CAD build for the part. Positions are in the model's coordinates, mm. A direction names the side the tool comes from. Give positions to 0.01 mm unless a question says otherwise; leave off trailing zeros. Order: outer loops, then holes, each group sorted by start corner. A loop starts at its lowest first (then second) coordinate and runs counter-clockwise, first axis right, second up. Notation, with made-up numbers: M -18.75,42.5 L 22.25,42.5 A9 cw 22.25,51.5 Z; hole C 78,59.25 d2. An arc over 180 degrees is marked long. Put each result on its own line as item: value. Start each with the question number.
1) Cut at A-A (z = -17). Write the cut outline in (x, y), and give its area (3 significant figures).
2) Cut at C-C (y = 4). Give the number of separate pieces and of enclosed holes in the cut face, and give its area (3 significant figures).
3) Cut at B-B (x = 14). Write the cut outline in (y, z), and give its area (3 significant figures).
4) Tool access for faces 1 (the face through (-6.8, 4.7, 12.9)), 2 (the face through (-12.9, 4.7, 6.8)), 3 (the face through (-15.5, 4.8, 12)), 4 (the face through (9.3, 4.8, -13.9)), 5 (the face through (12.6, 4.7, -6.8)): list every direction of +Z, -Z, +X, -X, +Y, -Y with a clear straight run to the whole face (end or side of a thin tool).
5) Pin check, flat tips, straight feed: pin 1 (1.5 mm diameter, centred on x = 15, z = 14.5, fed in from +Y); pin 2 (1 mm diameter, centred on y = 5, z = -11.5, fed in from -X); pin 3 (2.5 mm diameter, centred on y = 5.5, z = 19, fed in from -X). Stop position of each tip, or through.
6) Two-plate mould, pull along Z, no slides. Class faces 6 (the face through (-14, 3.5, 14)), 7 (the face through (18.7, 4.8, 14.1)), 8 (the face through (13.9, 4.8, -18.7)): released by +Z, released by -Z, zero draft, split by the parting line, or undercut.
7) Drill centre lines: line 1 (X direction, y = 4, z = -15); line 2 (Z direction, x = -12, y = 4.5); line 3 (Z direction, x = -10.5, y = 4.75). Where is each one in solid material? Low to high. Write a range as [from, to].
8) Cut at D-D (z = -12.5). Write the cut outline in (x, y), and give its area (3 significant figures).
```python
from build123d import *

# Parameters (mm, degrees)
SKETCH1_W               = 40
SKETCH1_H               = 40
BOSS_EXTRUDE1_DEPTH     = 6
SKETCH2_W               = 12
SKETCH2_H               = 12
CUT_EXTRUDE1_DEPTH      = 2.5
CHAMFER1_SIZE           = 2.5
SKETCH3_W               = 12
SKETCH3_H               = 12
BOSS_EXTRUDE2_DEPTH     = 2.5
CHAMFER2_SIZE           = 2.5
CIRPATTERN1_OUTLINE_W   = 7
CIRPATTERN1_OUTLINE_H   = 7
CIRPATTERN1_DEPTH       = 2.5
CIRPATTERN1_DRAFT       = 45
CIRPATTERN1_2_OUTLINE_W = 7
CIRPATTERN1_2_OUTLINE_H = 7
CIRPATTERN1_2_DEPTH     = 2.5
CIRPATTERN1_2_DRAFT     = 45
CIRPATTERN1_3_OUTLINE_W = 7
CIRPATTERN1_3_OUTLINE_H = 7
CIRPATTERN1_3_DEPTH     = 2.5
CIRPATTERN1_3_DRAFT     = 45
SKETCH4_R               = 2.5
CUT_EXTRUDE2_DEPTH      = 2.5
CIRPATTERN2_COUNT       = 4


# Read off the part's stored shape, not the designer's step: CirPattern1
# Some blends are built 0.0001 mm under size
with BuildPart() as part:
    # Sketch1 → Boss-Extrude1 (new body)
    with BuildSketch(Plane(origin=(0, 0, 0), x_dir=(1, 0, 0), z_dir=(0, 1, 0))):
        Rectangle(SKETCH1_W, SKETCH1_H)
    extrude(amount=BOSS_EXTRUDE1_DEPTH)

    # Sketch2 → Cut-Extrude1 (cut)
    with BuildSketch(Plane(origin=(0, 6, 0), x_dir=(1, 0, 0), z_dir=(0, 1, 0))):
        with Locations((14, 14)):
            Rectangle(SKETCH2_W, SKETCH2_H)
        with Locations((-14, 14)):
            Rectangle(SKETCH2_W, SKETCH2_H)
        with Locations((14, -14)):
            Rectangle(SKETCH2_W, SKETCH2_H)
        with Locations((-14, -14)):
            Rectangle(SKETCH2_W, SKETCH2_H)
    extrude(amount=-CUT_EXTRUDE1_DEPTH, mode=Mode.SUBTRACT)

    # Chamfer1
    chamfer1_edges = [part.edges().sort_by_distance(p)[0] for p in [
        (-20, 6, 0),
        (-14, 6, -8),
        (-8, 6, -14),
        (0, 6, -20),
        (8, 6, -14),
        (14, 6, -8),
        (20, 6, 0),
        (14, 6, 8),
        (8, 6, 14),
        (0, 6, 20),
        (-8, 6, 14),
        (-14, 6, 8),
    ]]
    chamfer(chamfer1_edges, length=CHAMFER1_SIZE - 0.0001)  # a hair under: the kernel refuses the full size

    # Sketch3 → Boss-Extrude2 (add)
    with BuildSketch(Plane(origin=(0, 3.5, 0), x_dir=(1, 0, 0), z_dir=(0, 1, 0))):
        with Locations((-14, -14)):
            Rectangle(SKETCH3_W, SKETCH3_H)
    extrude(amount=BOSS_EXTRUDE2_DEPTH)

    # Chamfer2
    # the kernel refuses this chamfer: 2.5 mm, written as the material it takes off along each edge
    with BuildSketch(Plane(origin=(-26.42920747, 6, 8), x_dir=(0, -0.9996219169112968, -0.027495876610586317), z_dir=(1, 0, 0)), Plane(origin=(-8, 6, 8), x_dir=(0.027495876610586317, -0.9996219169112968, 0), z_dir=(0, 0, 1))) as chamfer2_piece_1:
        Polygon((CHAMFER2_SIZE * 0.999621916911, -CHAMFER2_SIZE * 0.0274958766106), (-CHAMFER2_SIZE * 0.0274958766106, -CHAMFER2_SIZE * 0.999621916911), (0, 0), align=None)
    extrude(amount=18.42920747, mode=Mode.SUBTRACT)
    with BuildSketch(Plane(origin=(-1.57079253, 6, 20), x_dir=(0, -0.9996219169112968, 0.027495876610586317), z_dir=(-1, 0, 0))) as chamfer2_piece_2:
        Polygon((CHAMFER2_SIZE * 0.999621916911, -CHAMFER2_SIZE * 0.0274958766106), (-CHAMFER2_SIZE * 0.0274958766106, -CHAMFER2_SIZE * 0.999621916911), (0, 0), align=None)
    extrude(amount=24.85841494, mode=Mode.SUBTRACT)
    with BuildSketch(Plane(origin=(-20, 6, 26.42920747), x_dir=(0.9996219169112968, 0.027495876610586317, 0), z_dir=(0, 0, -1))) as chamfer2_piece_3:
        Polygon((CHAMFER2_SIZE * 0.999621916911, CHAMFER2_SIZE * 0.0274958766106), (-CHAMFER2_SIZE * 0.0274958766106, CHAMFER2_SIZE * 0.999621916911), (0, 0), align=None)
    extrude(amount=24.85841494, mode=Mode.SUBTRACT)


with BuildPart() as cirpattern1_tool:
    # CirPattern1 outline → CirPattern1 (with draft: the straight prism first)
    with BuildSketch(Plane(origin=(0, 6, 0), x_dir=(1, 0, 0), z_dir=(0, 1, 0))):
        with Locations((14, -14)):
            Rectangle(CIRPATTERN1_OUTLINE_W, CIRPATTERN1_OUTLINE_H)
    extrude(amount=-CIRPATTERN1_DEPTH)
    # CirPattern1: the draft: its side faces are tilted about the plane it starts from
    cirpattern1_sides = [cirpattern1_tool.faces().sort_by_distance(p)[0] for p in [
        (14, 4.75, 10.5),
        (10.5, 4.75, 14),
        (14, 4.75, 17.5),
        (17.5, 4.75, 14),
    ]]
    draft(cirpattern1_sides, Plane(origin=(0, 6, 0), x_dir=(1, 0, 0), z_dir=(0, 1, 0)), CIRPATTERN1_DRAFT)


with BuildPart() as part_1:
    add(part.part)

    # CirPattern1: add cirpattern1_tool
    add(cirpattern1_tool.part)


with BuildPart() as cirpattern1_2_tool:
    # CirPattern1 2 outline → CirPattern1 2 (with draft: the straight prism first)
    with BuildSketch(Plane(origin=(0, 6, 0), x_dir=(1, 0, 0), z_dir=(0, 1, 0))):
        with Locations((14, 14)):
            Rectangle(CIRPATTERN1_2_OUTLINE_W, CIRPATTERN1_2_OUTLINE_H)
    extrude(amount=-CIRPATTERN1_2_DEPTH)
    # CirPattern1 2: the draft: its side faces are tilted about the plane it starts from
    cirpattern1_2_sides = [cirpattern1_2_tool.faces().sort_by_distance(p)[0] for p in [
        (10.5, 4.75, -14),
        (14, 4.75, -10.5),
        (17.5, 4.75, -14),
        (14, 4.75, -17.5),
    ]]
    draft(cirpattern1_2_sides, Plane(origin=(0, 6, 0), x_dir=(1, 0, 0), z_dir=(0, 1, 0)), CIRPATTERN1_2_DRAFT)


with BuildPart() as part_2:
    add(part_1.part)

    # CirPattern1 2: add cirpattern1_2_tool
    add(cirpattern1_2_tool.part)


with BuildPart() as cirpattern1_3_tool:
    # CirPattern1 3 outline → CirPattern1 3 (with draft: the straight prism first)
    with BuildSketch(Plane(origin=(0, 6, 0), x_dir=(1, 0, 0), z_dir=(0, 1, 0))):
        with Locations((-14, 14)):
            Rectangle(CIRPATTERN1_3_OUTLINE_W, CIRPATTERN1_3_OUTLINE_H)
    extrude(amount=-CIRPATTERN1_3_DEPTH)
    # CirPattern1 3: the draft: its side faces are tilted about the plane it starts from
    cirpattern1_3_sides = [cirpattern1_3_tool.faces().sort_by_distance(p)[0] for p in [
        (-14, 4.75, -10.5),
        (-10.5, 4.75, -14),
        (-14, 4.75, -17.5),
        (-17.5, 4.75, -14),
    ]]
    draft(cirpattern1_3_sides, Plane(origin=(0, 6, 0), x_dir=(1, 0, 0), z_dir=(0, 1, 0)), CIRPATTERN1_3_DRAFT)


with BuildPart() as part_3:
    add(part_2.part)

    # CirPattern1 3: add cirpattern1_3_tool
    add(cirpattern1_3_tool.part)

    # Sketch4 → Cut-Extrude2 (cut)
    with BuildSketch(Plane(origin=(0, 6, 0), x_dir=(1, 0, 0), z_dir=(0, 1, 0))):
        with Locations(Location((-14, -14, 0), (0, 0, 270))):
            Circle(SKETCH4_R)
    cut_extrude2 = extrude(amount=-CUT_EXTRUDE2_DEPTH, mode=Mode.SUBTRACT)

    # CirPattern2: Cut-Extrude2 ×4 about axis
    cirpattern2_axis = Axis((0, 0, 0), (0, 1, 0))
    for i in range(1, CIRPATTERN2_COUNT):
        add(cut_extrude2.rotate(cirpattern2_axis, i * 360 / CIRPATTERN2_COUNT), mode=Mode.SUBTRACT)


solid = part_3.part
```
Solution:
1. outline: M -20,0 L 20,0 L 20,3.5 L 17.5,6 L 10.5,6 L 8,3.5 L 5.5,6 L -5.5,6 L -8,3.5 L -10.5,6 L -17.5,6 L -20,3.5 Z
1. area: 221 mm²
2. separate pieces: 5
2. enclosed holes: 4
2. area: 1,350 mm²
3. outline: M 0,-20 L 3.5,-20 L 6,-17.5 L 6,-16.5 L 3.5,-16.5 L 3.5,-11.5 L 6,-11.5 L 6,-10.5 L 3.5,-8 L 6,-5.5 L 6,5.5 L 3.5,8 L 6,10.5 L 6,11.5 L 3.5,11.5 L 3.5,16.5 L 6,16.5 L 6,17.5 L 3.5,20 L 0,20 Z
3. area: 196 mm²
4. face 1: +Z, +Y
4. face 2: -X, +Y
4. face 3: +Y
4. face 4: -Z, +Y
4. face 5: +X, +Y
5. pin 1: y = 3.5
5. pin 2: x = -19
5. pin 3: x = -19.25
6. face 6: undercut
6. face 7: zero draft
6. face 8: released by -Z
7. line 1: [-19.5, -16.29], [-11.71, -8.5], [-7.5, 7.5], [8.5, 11.71], [16.29, 19.5]
7. line 2: [-19, -15.5], [-12.5, -9], [-7, 7], [9, 12.5], [15.5, 19]
7. line 3: [-18.75, -9.25], [-6.75, 6.75], [9.25, 18.75]
8. outline: M -20,0 L 20,0 L 20,3.5 L 17.5,6 L 16,6 L 16,3.5 L 12,3.5 L 12,6 L 10.5,6 L 8,3.5 L 5.5,6 L -5.5,6 L -8,3.5 L -10.5,6 L -12,6 L -12,3.5 L -16,3.5 L -16,6 L -17.5,6 L -20,3.5 Z
8. area: 201 mm²
